The drawing under review shows one solid part. Ordinate dimensions are in mm from its lowest x, y, z. A direction names the side the tool comes from. Give positions to 0.01 mm unless a question says otherwise; leave off trailing zeros. Order: outer loops, then holes, each group sorted by start corner. A loop starts at its lowest first (then second) coordinate and runs counter-clockwise, first axis right, second up. Notation, with made-up numbers: (76, -34) -> (130, -34) arc R17 cw to (130, -21) -> close; hole circle Ø4 at (56, -27). An arc over 180 degrees is marked (long way). Return JSON: item names as keys, results as strings. Group by question number.
1) For the marked faces 1, 2 and 3, list the 3-axis set-ups (+Z, -Z, +X, -X, +Y, -Y) from which the entire face can be reached by the end or side of a thin tool; tool diameter is ignored.
2) Add section D-D (z = 5.75). Give the boundary of the cut face in (x, y).
3) To check wall thickness, follow line 1 along Y through (x, z) = (23, 2.25); line 2 along X through (y, z) = (27, 9.75); line 3 along Y through (x, z) = (25, 20.5). State the ranges of each line that lie inside material, in increasing order.
4) Insertion check: P1, Ø1, axis at y = 59, z = 5.5, coming from the +X side; P2, Ø0.8, axis at x = 28, y = 59, coming from the +Z side; P3, Ø1.5, axis at x = 5.5, z = 13.5, coming from the +Y side; P4, Ø2.5, axis at y = 31, z = 19.775, coming from the -X side. Each pin has a flat end and moves straight along its axis. Give the tip position at first contact, or say it passes through.
5) Add section C-C (y = 11.5). Give the boundary of the cut face in (x, z).
6) Add section A-A (y = 31). Give the boundary of the cut face in (x, z) (3 decimals), then the cut area to 3 significant figures.
7) Add section B-B (z = 11). Give the boundary of the cut face in (x, y).
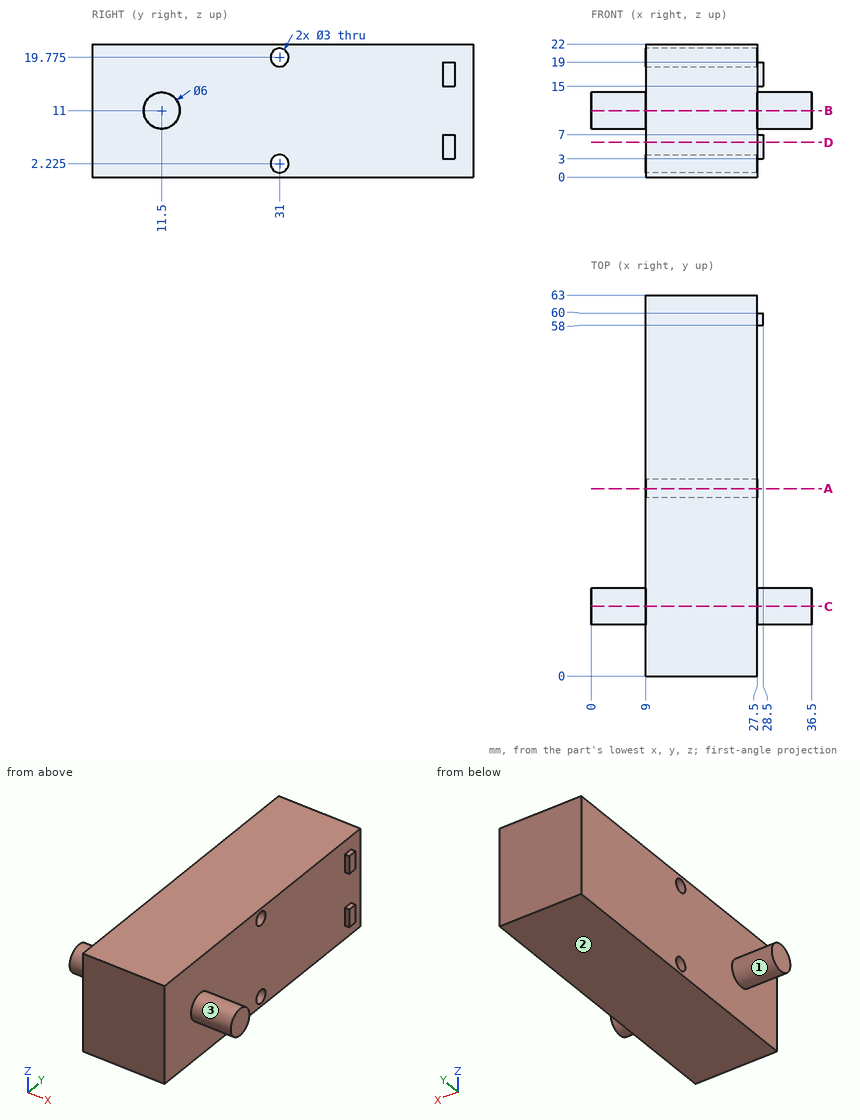
Evaluation:
{
 "1": {"face 1": "-X", "face 2": "-Z, +X, -X, +Y, -Y", "face 3": "+X"},
 "2": {"outline": "(9, 0) -> (27.5, 0) -> (27.5, 58) -> (28.5, 58) -> (28.5, 60) -> (27.5, 60) -> (27.5, 63) -> (9, 63) -> close"},
 "3": {"line 1": "0 to 29.5, 32.5 to 63", "line 2": "9 to 27.5", "line 3": "0 to 29.69, 32.31 to 63"},
 "4": {"P1": "x = 28.5", "P2": "z = 19", "P3": "y = 13.94", "P4": "through"},
 "5": {"outline": "(0, 8) -> (9, 8) -> (9, 0) -> (27.5, 0) -> (27.5, 8) -> (36.5, 8) -> (36.5, 14) -> (27.5, 14) -> (27.5, 22) -> (9, 22) -> (9, 14) -> (0, 14) -> close"},
 "6": {"outline": "(9, 0) -> (27.5, 0) -> (27.5, 0.725) -> (9, 0.725) -> close; (9, 3.725) -> (27.5, 3.725) -> (27.5, 18.275) -> (9, 18.275) -> close; (9, 21.275) -> (27.5, 21.275) -> (27.5, 22) -> (9, 22) -> close", "area": "296 mm^2"},
 "7": {"outline": "(0, 8.5) -> (9, 8.5) -> (9, 0) -> (27.5, 0) -> (27.5, 8.5) -> (36.5, 8.5) -> (36.5, 14.5) -> (27.5, 14.5) -> (27.5, 63) -> (9, 63) -> (9, 14.5) -> (0, 14.5) -> close"}
}
